from build123d import *

# Parameters (mm, degrees)
WALL_EXTRUDE_DEPTH           = 200
RIGHT_GUIDE_EXTRUDE_DEPTH    = 10
SKETCH3_W                    = 600
SKETCH3_H                    = 210
BOTTOM_FOOT_COMPLETION_DEPTH = 10
SKETCH4_W                    = 400
SKETCH4_H                    = 10
PLATFORM_STOPPER_DEPTH       = 28
STRUCTURAL_FILLETS_R         = 10


with BuildPart() as part:
    # Sketch1 → Wall extrude (new, symmetric)
    with BuildSketch(Plane(origin=(0, 0, 0), x_dir=(0, 0, -1), z_dir=(1, 0, 0))):
        Polygon((0, 0), (-100, 0), (-100, -10), (10, -10), (110, -10), (110, 0), (10, 0), (10, 1741.5), (0, 1741.5), align=None)
    extrude(amount=WALL_EXTRUDE_DEPTH, both=True)

    # Sketch2 → Right guide extrude (add)
    with BuildSketch(Plane(origin=(200, 0, 0), x_dir=(0, 0, -1), z_dir=(1, 0, 0))):
        Polygon((0, 1741.5), (38, 1741.5), (38, -10), (0, -10), (-28, -10), (-28, 1741.5), align=None)
        with BuildLine():
            Line((18, 226.5), (18, 1726.5))
            ThreePointArc((18, 1726.5), (23, 1731.5), (28, 1726.5))
            Line((28, 1726.5), (28, 226.5))
            ThreePointArc((28, 226.5), (23, 221.5), (18, 226.5))
        make_face(mode=Mode.SUBTRACT)
        with BuildLine():
            Line((-18, 1726.5), (-18, 226.5))
            ThreePointArc((-18, 226.5), (-13, 221.5), (-8, 226.5))
            Line((-8, 226.5), (-8, 1726.5))
            ThreePointArc((-8, 1726.5), (-13, 1731.5), (-18, 1726.5))
        make_face(mode=Mode.SUBTRACT)
    right_guide_extrude = extrude(amount=RIGHT_GUIDE_EXTRUDE_DEPTH)

    # Left guide extrude: Right guide extrude across plane
    add(right_guide_extrude.mirror(Plane(origin=(0, 0, 0), x_dir=(0, 0, 1), z_dir=(1, 0, 0))))

    # Sketch3 → Bottom foot completion (add)
    with BuildSketch(Plane.XZ.offset(10)):
        with Locations((0, -5)):
            Rectangle(SKETCH3_W, SKETCH3_H)
    extrude(amount=-BOTTOM_FOOT_COMPLETION_DEPTH)

    # Sketch4 → Platform stopper (add)
    with BuildSketch(Plane(origin=(0, 0, -10), x_dir=(-1, 0, 0), z_dir=(0, 0, -1))):
        with Locations((0, 131.5)):
            Rectangle(SKETCH4_W, SKETCH4_H)
    extrude(amount=PLATFORM_STOPPER_DEPTH)

    # Structural fillets
    structural_fillets_edges = [part.edges().sort_by_distance(p)[0] for p in [
        (205, 0, 28),
        (205, 0, -38),
        (210, 0, -5),
        (-205, 0, -38),
        (-210, 0, -5),
        (-205, 0, 28),
        (-200, 0, 14),
        (-200, 126.5, -24),
        (200, 126.5, -24),
        (0, 126.5, -10),
        (0, 0, -10),
        (0, 0, 0),
        (200, 0, -24),
        (-200, 0, -24),
        (200, 0, 14),
    ]]
    fillet(structural_fillets_edges, radius=STRUCTURAL_FILLETS_R)


solid = part.part
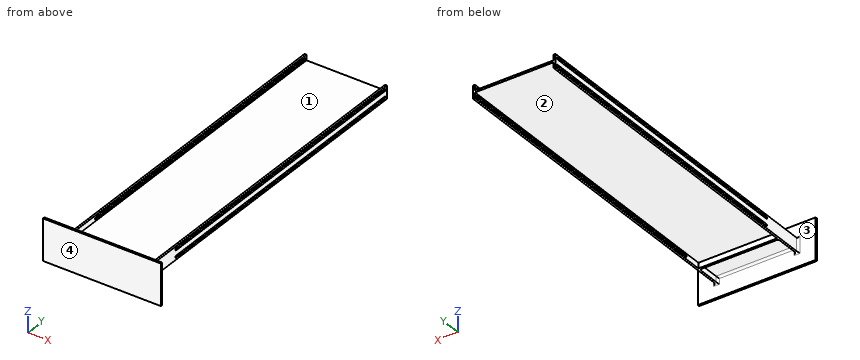
For this review, take the finished solid that the model builds, in its own axes (mm). Face numbers are marked on the shaded views. A direction names the side the tool comes from. Give positions to 0.01 mm unless a question says otherwise; leave off trailing zeros. Loops run counter-clockwise (first coordinate to the right, second up) from the corner with the lowest first, then second, coordinate; pieces in that order, holes last. Notation, with made-up numbers: (72.5, -28.5) - (89.5, -28.5) arc R13 ccw to (89.5, -6.5) - close; hole circle Ø10 at (2, 87). An arc over 180 degrees is marked (long way). Write each question's results on one line, items separated by ' | '.
(1) For line 1 along Z through (x, y) = (-209, 1224); line 2 along Y through (x, z) = (-65, -77.5), list the stretches that pass through material, from the lowest coordinate up.
Conclusion:
line 1: -38 to -28, -18 to 8, 18 to 28 | line 2: -10 to 0
(2) Take a section at B-B (z = -73). Give the boundary of the cut face in (x, y), then the cut area to 3 significant figures.
Conclusion:
outline: (-300, -10) - (300, -10) - (300, 0) - (-300, 0) - close | area: 6,000 mm^2
(3) For pin 1 Ø8 at (x, y) = (203.5, 1265) entering from +Z; pin 2 Ø14 at (y, z) = (65.5, -21.5) entering from +X; pin 3 Ø1 at (x, z) = (-90.5, 6) entering from +Y, all flat-tipped, find the tip position at first contact; note any pin that passes through.
Conclusion:
pin 1: z = 28 | pin 2: x = 210 | pin 3: y = 1.07
(4) Take a section at A-A (y = 1201). Give the boundary of the cut face in (x, z).
Conclusion:
outline: (-210, -38) - (-200, -38) - (-200, -28) - (-210, -28) - close; (-210, -18) - (-200, -18) - (-200, -10) - (200, -10) - (200, -18) - (210, -18) - (210, 8) - (200, 8) - (200, 0) - (-200, 0) - (-200, 8) - (-210, 8) - close; (-210, 18) - (-200, 18) - (-200, 28) - (-210, 28) - close; (200, -38) - (210, -38) - (210, -28) - (200, -28) - close; (200, 18) - (210, 18) - (210, 28) - (200, 28) - close
(5) For the marked faces 1 and 2, list the 3-axis set-ups (+Z, -Z, +X, -X, +Y, -Y) from which the entire face can be reached by the end or side of a thin tool; tool diameter is ignored.
Conclusion:
face 1: +Z, +Y | face 2: -Z, +Y
(6) Draft analysis for pull direction X (two halves, no side actions). For the marked faces 3 and 4, state which applies: +X half, -X half, draft (parallel to the pull), parting line (faces both ways), or undercut.
Conclusion:
face 3: undercut | face 4: draft
